from build123d import *

# Parameters (mm, degrees)
SKETCH1_W           = 127
SKETCH1_H           = 88.9
BOSS_EXTRUDE1_DEPTH = 31.75
SHELL1_T            = -2.54
SKETCH3_R           = 3.175
CUT_EXTRUDE2_DEPTH  = 31.75
SKETCH4_W           = 38.1
SKETCH4_H           = 26.035
CUT_EXTRUDE3_DEPTH  = 2.54
SKETCH5_W           = 25.4
SKETCH5_H           = 26.035
CUT_EXTRUDE4_DEPTH  = 2.54
SKETCH6_W           = 25.4
SKETCH6_H           = 63.5
CUT_EXTRUDE5_DEPTH  = 2.54


with BuildPart() as part:
    # Sketch1 → Boss-Extrude1 (new body)
    with BuildSketch(Plane(origin=(0, 0, 0), x_dir=(1, 0, 0), z_dir=(0, 1, 0))):
        with Locations((63.5, 44.45)):
            Rectangle(SKETCH1_W, SKETCH1_H)
    extrude(amount=BOSS_EXTRUDE1_DEPTH)

    # Shell1
    shell1_openings = [part.faces().sort_by_distance(p)[0] for p in [
        (63.5, 31.75, -44.45),
    ]]
    offset(amount=SHELL1_T, openings=shell1_openings, kind=Kind.INTERSECTION)

    # Sketch3 → Cut-Extrude2 (cut)
    with BuildSketch(Plane(origin=(127, 0, 0), x_dir=(0, 0, -1), z_dir=(1, 0, 0))):
        with Locations((12.7, 25.4)):
            Circle(SKETCH3_R)
        with Locations((76.2, 25.4)):
            Circle(SKETCH3_R)
    cut_extrude2 = extrude(amount=-CUT_EXTRUDE2_DEPTH, mode=Mode.SUBTRACT)

    # Mirror2: Cut-Extrude2 across plane
    add(cut_extrude2.mirror(Plane(origin=(63.5, 0, 0), x_dir=(0, 0, 1), z_dir=(1, 0, 0))), mode=Mode.SUBTRACT)

    # Sketch4 → Cut-Extrude3 (cut)
    with BuildSketch(Plane(origin=(0, 0, -88.9), x_dir=(-1, 0, 0), z_dir=(0, 0, -1))):
        with Locations((-99.06, 18.7325)):
            Rectangle(SKETCH4_W, SKETCH4_H)
    extrude(amount=-CUT_EXTRUDE3_DEPTH, mode=Mode.SUBTRACT)

    # Sketch5 → Cut-Extrude4 (cut)
    with BuildSketch(Plane.XY):
        with Locations((53.34, 18.7325)):
            Rectangle(SKETCH5_W, SKETCH5_H)
    extrude(amount=-CUT_EXTRUDE4_DEPTH, mode=Mode.SUBTRACT)

    # Sketch6 → Cut-Extrude5 (cut)
    with BuildSketch(Plane.XZ):
        with Locations((99.06, -40.64)):
            Rectangle(SKETCH6_W, SKETCH6_H)
    extrude(amount=-CUT_EXTRUDE5_DEPTH, mode=Mode.SUBTRACT)


solid = part.part
Read the model definition and answer for the solid it produces. Units are mm, in the model's axes. A direction names the side the tool comes from. Give positions to 0.01 mm unless a question says otherwise; leave off trailing zeros. Write each loop counter-clockwise with the first axis right and the second up, starting at its lowest first coordinate (ties: lowest second). Pieces come first, ordered by that corner, then holes. Notation, with made-up numbers: (42, -1) - (101, -1) arc R10 ccw to (101, 5) - close; hole circle Ø10 at (43, 48.5). An arc over 180 degrees is marked (long way). Use CSV: the item, a comma, the result in double quotes. Start each with the question number.
(1) Find section A-A (z = -76.2). Give the vertices of the cut face in (x, y) (3 decimals), plus the area to 3 significant figures.
(2) Find section D-D (z = -12.7). Give the vertices of the cut face in (x, y) (3 decimals), plus the area to 3 significant figures.
(3) Determine the mould class of faces 4 (the flat face through (63, 0, -45)), 5 (the flat face through (49, 17, -86.36)), 6 (the cylindrical face through (1.25, 28.55, -12.29)) for opening direction Y: +Y half, -Y half, draft (parallel to the pull), parting line (faces both ways), or undercut.
(4) Find section B-B (y = 19.5). Give the vertices of the cut face in (x, z).
(5) Find section C-C (x = 95). Give the vertices of the cut face in (y, z) (3 decimals), plus the area to 3 significant figures.
(6) For faces 1 (the flat face through (118.11, 19, -88)), 2 (the flat face through (99, 1, -72.39)), 3 (the flat face through (124.46, 17, -44)), determine the directions among +Z, -Z, +X, -X, +Y, -Y from which every point of the face is accessible in a straight line to the end or side of a thin tool.
(7) Given P1, Ø1.3, axis at x = 56.5, z = -1.5, coming from the +Y side (3 decimals); P2, Ø1, axis at x = 13.5, z = -68.5, coming from the +Y side, each flat-ended and moving along its own axis, determine where each tip first touches the part or whether it passes through.
(8) Consider line 1 along Z through (x, y) = (1.4, 25.4) (3 decimals); line 2 along Z through (x, y) = (120.5, 7.5); line 3 along X through (y, z) = (20.5, -19). Determine where each line is inside the solid, lowest interval first.
Findings below:
1,outline,"(0, 0) - (127, 0) - (127, 22.225) - (124.46, 22.225) - (124.46, 2.54) - (2.54, 2.54) - (2.54, 22.225) - (0, 22.225) - close; (0, 28.575) - (2.54, 28.575) - (2.54, 31.75) - (0, 31.75) - close; (124.46, 28.575) - (127, 28.575) - (127, 31.75) - (124.46, 31.75) - close"
1,area,"439 mm2"
2,outline,"(0, 0) - (86.36, 0) - (86.36, 2.54) - (2.54, 2.54) - (2.54, 22.225) - (0, 22.225) - close; (0, 28.575) - (2.54, 28.575) - (2.54, 31.75) - (0, 31.75) - close; (111.76, 0) - (127, 0) - (127, 22.225) - (124.46, 22.225) - (124.46, 2.54) - (111.76, 2.54) - close; (124.46, 28.575) - (127, 28.575) - (127, 31.75) - (124.46, 31.75) - close"
2,area,"374 mm2"
3,face 4,"-Y half"
3,face 5,"draft"
3,face 6,"undercut"
4,outline,"(0, -88.9) - (80.01, -88.9) - (80.01, -86.36) - (2.54, -86.36) - (2.54, -2.54) - (40.64, -2.54) - (40.64, 0) - (0, 0) - close; (66.04, -2.54) - (124.46, -2.54) - (124.46, -86.36) - (118.11, -86.36) - (118.11, -88.9) - (127, -88.9) - (127, 0) - (66.04, 0) - close"
5,outline,"(0, -88.9) - (5.715, -88.9) - (5.715, -86.36) - (2.54, -86.36) - (2.54, -72.39) - (0, -72.39) - close; (0, -8.89) - (2.54, -8.89) - (2.54, -2.54) - (31.75, -2.54) - (31.75, 0) - (0, 0) - close"
5,area,"147 mm2"
6,face 1,"-Z, +Y"
6,face 2,"+Y, -Y"
6,face 3,"+Y"
7,P1,"y = 5.715"
7,P2,"y = 2.54"
8,line 1,"-88.9 to -79.375, -73.025 to -15.875, -9.525 to 0"
8,line 2,"-88.9 to -86.36, -2.54 to 0"
8,line 3,"0 to 2.54, 124.46 to 127"
